Part print with two shaded views. Sizes in mm from the minimum x, y, z corner. Coordinates: 2 decimals unless noted, no trailing zeros. Write each loop counter-clockwise with the first axis right and the second up, starting at its lowest first coordinate (ties: lowest second). Pieces come first, ordered by that corner, then holes. Notation, with made-up numbers: M -15.5,86.25 L 11.5,86.25 A26 ccw 11.5,121.25 Z; hole C 34.5,57.5 d10. An arc over 180 degrees is marked long. One line per question, with ' | ' between items. Start each with the question number.
(1) Flat gauge pins, fed straight in: pin 1 Ø4 at (x, z) = (56, 6) entering from -Y; pin 2 Ø6 at (x, z) = (28, 6) entering from -Y; pin 3 Ø1.5 at (x, z) = (45.5, 3) entering from +Y. Where does each tip first touch, or does it go through?
(2) Wall check: probe 1 along X at (y, z) = (6, 6); probe 2 along Z at (x, y) = (28, 11); probe 3 along X at (y, z) = (8.75, 10). Give the ranges that are in metal, low to high.
(3) Cut at D-D (z = 5). Count the separate pieces of the cut face and the enclosed holes in it, plus the area to 3 significant figures.
(4) Cut at B-B (x = 56). Write the cut outline in (y, z).
(5) Cut at C-C (x = 70). Write the cut outline in (y, z), plus the area to 3 significant figures.
(6) Cut at A-A (y = 8.5). Write the cut outline in (x, z), plus the area to 3 significant figures.
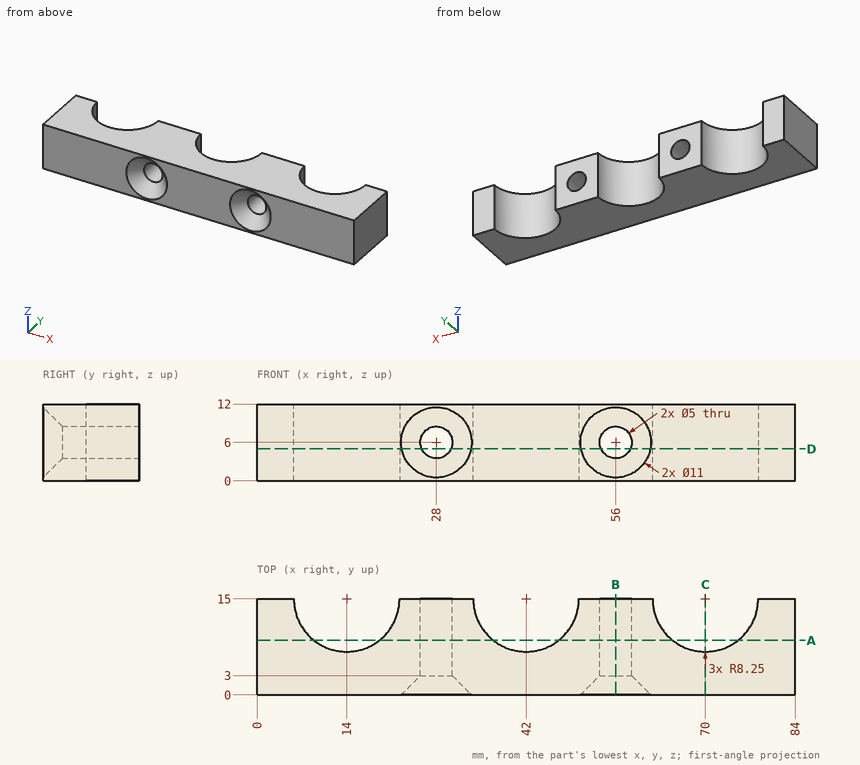
Filled in:
1) pin 1: through | pin 2: y = 2.5 | pin 3: y = 7.93
2) probe 1: 0 to 25.5, 30.5 to 53.5, 58.5 to 84 | probe 2: 0 to 3.5, 8.5 to 12 | probe 3: 0 to 8.61, 19.39 to 36.61, 47.39 to 64.61, 75.39 to 84
3) separate pieces: 3 | enclosed holes: 0 | area: 783 mm²
4) outline: M 0,0 L 15,0 L 15,3.5 L 3,3.5 L 0,0.5 Z; M 0,11.5 L 3,8.5 L 15,8.5 L 15,12 L 0,12 Z
5) outline: M 0,0 L 6.75,0 L 6.75,12 L 0,12 Z | area: 81.0 mm²
6) outline: M 0,0 L 8.92,0 L 8.92,12 L 0,12 Z; M 19.08,0 L 36.92,0 L 36.92,12 L 19.08,12 Z; M 47.08,0 L 64.92,0 L 64.92,12 L 47.08,12 Z; M 75.08,0 L 84,0 L 84,12 L 75.08,12 Z; hole C 28,6 d5; hole C 56,6 d5 | area: 603 mm²
